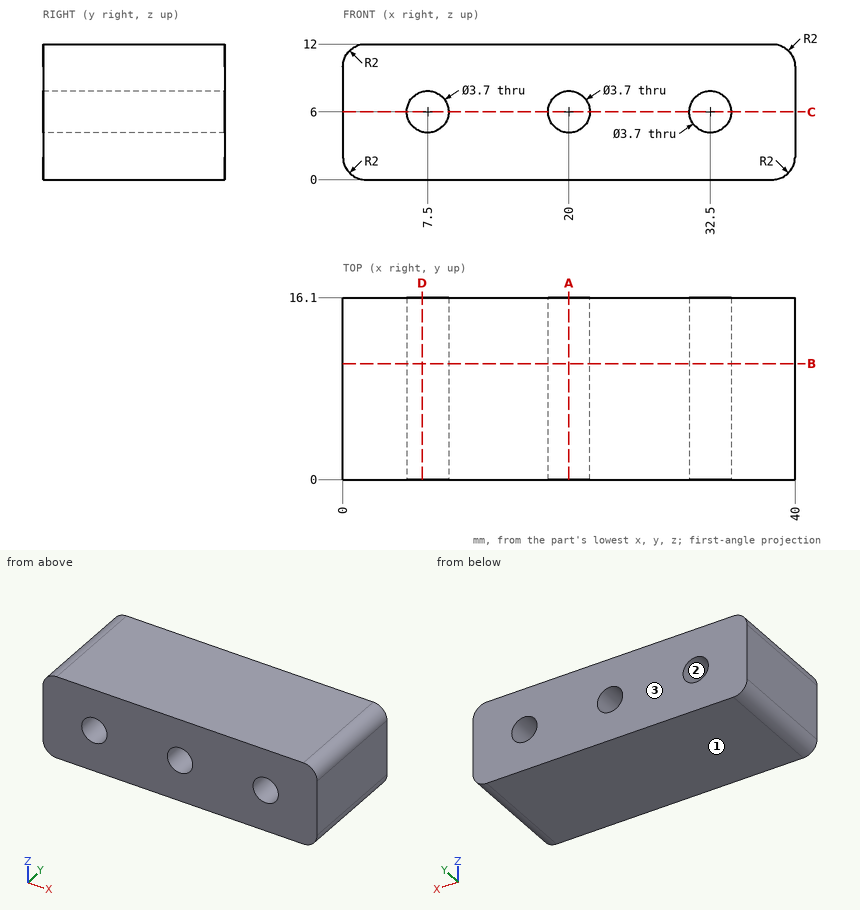
Geometry: see drawing. Coordinates: mm, zero at the bounding-box minimum. Give positions to 0.01 mm unless a question says otherwise; leave off trailing zeros. Write each loop counter-clockwise with the first axis right and the second up, starting at its lowest first coordinate (ties: lowest second). Pieces come first, ordered by that corner, then holes. Notation, with made-up numbers: M -25,43.25 L 23,43.25 A34 cw 23,78.25 Z; hole C -22.5,46 d6. An arc over 180 degrees is marked long. Answer in a Markdown table with one row per item. Add a question column.
(1) Section B-B on y = 10.25. Return loops of the section in (x, z).
(2) Section C-C on z = 6. Return loops of the section in (x, y), and give its area (3 significant figures).
(3) Mould query, pull axis Z, two halves, no side actions, for the marked faces 1, 2 and 3. Classes: +Z half, -Z half, draft (parallel to the pull), parting line (faces both ways), or undercut.
(4) First-contact query: pin 1 (3 mm diameter, centred on x = 32.5, z = 6, fed in from +Y). Flat tip, straight axial feed; report the tip coordinate or a pass-through.
(5) Section D-D on x = 7. Return loops of the section in (y, z).
(6) Section A-A on x = 20. Return loops of the section in (y, z), and give its area (3 significant figures).
(7) Ray query, line 1 (X direction, y = 7.25, z = 6); line 2 (X direction, y = 6.5, z = 7); line 3 (Z direction, x = 21, y = 6). Return the intervals inside material, ascending.
Result set:
| question | item | result |
|---|---|---|
| 1 | outline | M 0,2 A2 ccw 2,0 L 38,0 A2 ccw 40,2 L 40,10 A2 ccw 38,12 L 2,12 A2 ccw 0,10 Z; hole C 7.5,6 d3.7; hole C 20,6 d3.7; hole C 32.5,6 d3.7 |
| 2 | outline | M 0,0 L 5.65,0 L 5.65,16.1 L 0,16.1 Z; M 9.35,0 L 18.15,0 L 18.15,16.1 L 9.35,16.1 Z; M 21.85,0 L 30.65,0 L 30.65,16.1 L 21.85,16.1 Z; M 34.35,0 L 40,0 L 40,16.1 L 34.35,16.1 Z |
| 2 | area | 465 mm^2 |
| 3 | face 1 | -Z half |
| 3 | face 2 | undercut |
| 3 | face 3 | draft |
| 4 | pin 1 | passes through |
| 5 | outline | M 0,0 L 16.1,0 L 16.1,4.22 L 0,4.22 Z; M 0,7.78 L 16.1,7.78 L 16.1,12 L 0,12 Z |
| 6 | outline | M 0,0 L 16.1,0 L 16.1,4.15 L 0,4.15 Z; M 0,7.85 L 16.1,7.85 L 16.1,12 L 0,12 Z |
| 6 | area | 134 mm^2 |
| 7 | line 1 | x = 0 to 5.65, 9.35 to 18.15, 21.85 to 30.65, 34.35 to 40 |
| 7 | line 2 | x = 0 to 5.94, 9.06 to 18.44, 21.56 to 30.94, 34.06 to 40 |
| 7 | line 3 | z = 0 to 4.44, 7.56 to 12 |
